Read the model definition and answer for the solid it produces. Units are mm, in the model's axes. A direction names the side the tool comes from. Round coordinates to 2 decimals unless told otherwise and drop trailing zeros. Order: outer loops, then holes, each group sorted by start corner. A loop starts at its lowest first (then second) coordinate and runs counter-clockwise, first axis right, second up. Notation, with made-up numbers: (7, 2) - (45, 2) arc R33 cw to (45, 38) - close; hole circle Ø7 at (27, -13.75). An arc over 180 degrees is marked (long way). Answer as a JSON object with one key per item and string values. Group by question number.
Q1. A cutting plane is placed at B-B on z = -11. Determine the outline of the cut face in (x, y), and give its area (3 significant figures).
Q2. A tool of negligible diameter and unlimited length cuts with its end or side. For faces 4 (the flat face through (-20, -5, 4.853)), 5 (the flat face through (-12.155, -5, -23)), 6 (the flat face through (16, -5, 19.077)), 7 (the flat face through (21, -5, -5.815)), from which of +Z, -Z, +X, -X, +Y, -Y can it reach the whole face along a straight path? Write none if from no direction.
Q3. Consider line 1 (Z direction, x = 20, y = -2.75); line 2 (X direction, y = -9.5, z = -22); line 3 (X direction, y = -8, z = -18.5). Determine where each line is inside the solid, lowest interval first.
Q4. Given pin 1 Ø1.6 at (x, y) = (-20, -6) entering from +Z; pin 2 Ø1.6 at (x, y) = (-21, -7) entering from -Z; pin 3 Ø3 at (x, y) = (16.5, -6) entering from +Z, each flat-ended and moving along its own axis, determine where each tip first touches the part or whether it passes through.
Q5. A cutting plane is placed at A-A on z = 21.5. Determine the outline of the cut face in (x, y), and give its area (3 significant figures).
Q6. The mould has two halves that part along Z. Classify faces 1 (the flat face through (-22.061, -5, -8)), 2 (the flat face through (-20, -5, -16.483)), 3 (the flat face through (19.468, -5, 3)): pulls with the +Z half, pulls with the -Z half, needs draft (parallel to the pull), parting line crosses it, or undercut.
```python
from build123d import *

# Parameters (mm, degrees)
F1_DEPTH = 10.16


with BuildPart() as f1:
    # F0 (on Front) → F1 (new body)
    with BuildSketch(Plane.XZ):
        Polygon((-18.885527, -19.996368), (-12.154527, -20.039365), (-12.154527, -26.389365), (-8.598527, -26.389365), (-8.598527, -20.039365), (-5.042527, -20.039365), (-5.042527, -26.389365), (-1.486527, -26.389365), (-1.486527, -20.039365), (2.069473, -20.039365), (2.069473, -26.389365), (5.625473, -26.389365), (5.625473, -20.039365), (9.181473, -20.039365), (9.181473, -26.389365), (12.737473, -26.389365), (12.737473, -20.039365), (19.468473, -20.039365), (19.468473, -16.483365), (22.643473, -16.483365), (22.643473, -12.927365), (19.468473, -12.927365), (19.468473, -9.371365), (22.643473, -9.371365), (22.643473, -5.815365), (19.468473, -5.815365), (19.468473, -2.259365), (22.643473, -2.259365), (22.643473, 1.296635), (19.468473, 1.296635), (19.468473, 4.852635), (22.643473, 4.852635), (22.643473, 8.408635), (19.468473, 8.408635), (19.468473, 11.964635), (22.643473, 11.964635), (22.643473, 15.520635), (19.468473, 15.520635), (19.468473, 19.076635), (12.737473, 19.076635), (12.737473, 25.426635), (9.181473, 25.426635), (9.181473, 19.076635), (5.625473, 19.076635), (5.625473, 25.426635), (2.069473, 25.426635), (2.069473, 19.076635), (-1.486527, 19.076635), (-1.486527, 25.426635), (-5.042527, 25.426635), (-5.042527, 19.076635), (-8.598527, 19.076635), (-8.598527, 25.426635), (-12.154527, 25.426635), (-12.154527, 19.076635), (-18.885527, 19.076635), (-18.885527, 15.520635), (-22.060527, 15.520635), (-22.060527, 11.964635), (-18.885527, 11.964635), (-18.885527, 8.408635), (-22.060527, 8.408635), (-22.060527, 4.852635), (-18.885527, 4.852635), (-18.885527, 1.296635), (-22.060527, 1.296635), (-22.060527, -2.259365), (-18.885527, -2.259365), (-18.885527, -5.815365), (-22.060527, -5.815365), (-22.060527, -9.371365), (-18.885527, -9.371365), (-18.885527, -12.927365), (-22.060527, -12.927365), (-22.060527, -16.483365), (-18.885527, -16.483365), align=None)
    extrude(amount=F1_DEPTH)


solid = f1.part
```
Result set:
{
 "1": {"outline": "(-18.89, -10.16) - (19.47, -10.16) - (19.47, 0) - (-18.89, 0) - close", "area": "390 mm²"},
 "2": {"face 4": "-X, +Y, -Y", "face 5": "-Z, -X, +Y, -Y", "face 6": "+Z, +X, +Y, -Y", "face 7": "+X, +Y, -Y"},
 "3": {"line 1": "z = -16.48 to -12.93, -9.37 to -5.82, -2.26 to 1.3, 4.85 to 8.41, 11.96 to 15.52", "line 2": "x = -12.15 to -8.6, -5.04 to -1.49, 2.07 to 5.63, 9.18 to 12.74", "line 3": "x = -18.89 to 19.47"},
 "4": {"pin 1": "stops at z = 15.52", "pin 2": "stops at z = -16.48", "pin 3": "stops at z = 19.08"},
 "5": {"outline": "(-12.15, -10.16) - (-8.6, -10.16) - (-8.6, 0) - (-12.15, 0) - close; (-5.04, -10.16) - (-1.49, -10.16) - (-1.49, 0) - (-5.04, 0) - close; (2.07, -10.16) - (5.63, -10.16) - (5.63, 0) - (2.07, 0) - close; (9.18, -10.16) - (12.74, -10.16) - (12.74, 0) - (9.18, 0) - close", "area": "145 mm²"},
 "6": {"face 1": "needs draft", "face 2": "pulls with the -Z half", "face 3": "undercut"}
}
